The figure shows three views and two pictorial views of one solid part (mm, origin at its lowest corner). Answer the questions. A direction names the side the tool comes from. Round coordinates to 2 decimals unless told otherwise and drop trailing zeros. Write each loop counter-clockwise with the first axis right and the second up, starting at its lowest first coordinate (ties: lowest second). Pieces come first, ordered by that corner, then holes. Notation, with made-up numbers: (55, 70.5) -> (86, 70.5) arc R33 cw to (86, 106.5) -> close; hole circle Ø10 at (-21.5, 25). An arc over 180 degrees is marked (long way). One line per item, written item: value.
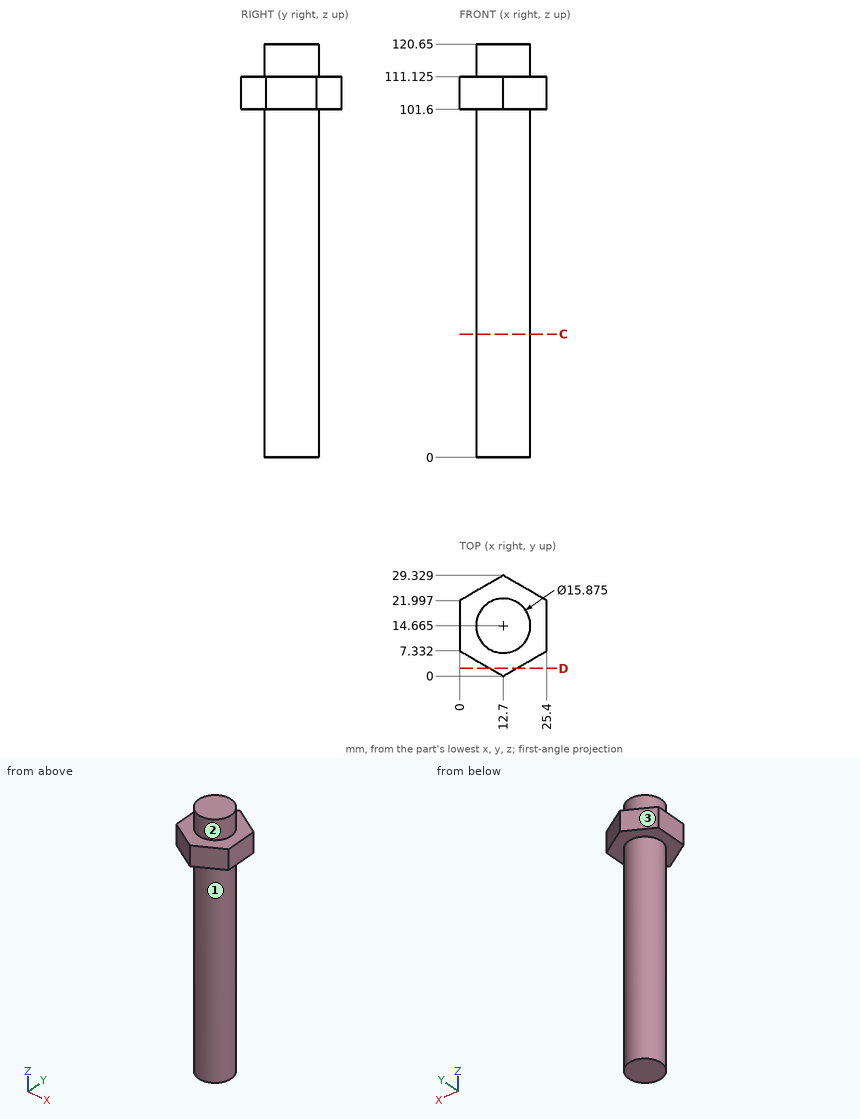
(1) Find section D-D on y = 2.25. Give the vertices of the cut face in (x, z) (1 decimal).
Reported:
outline: (8.8, 101.6) -> (16.6, 101.6) -> (16.6, 111.1) -> (8.8, 111.1) -> close
(2) Flat-ended cylindrical pins translate along their axes: pin 1 Ø7.5 at (x, y) = (18.5, 21.5) entering from -Z; pin 2 Ø1 at (x, z) = (7.5, 22.5) entering from -Y; pin 3 Ø4 at (x, y) = (4, 26) entering from -Z; pin 4 Ø2 at (y, z) = (12, 30) entering from +X. Find the tip coordinate at first contact, or state that the pin passes through.
Reported:
pin 1: stops at z = 0
pin 2: stops at y = 8.27
pin 3: stops at z = 101.6
pin 4: stops at x = 20.46
(3) A tool of negligible diameter and unlimited length cuts with its end or side. For the marked faces 1, 2 and 3, from which of +Z, -Z, +X, -X, +Y, -Y can it reach the whole face along a straight path? Write none if from no direction.
Reported:
face 1: -Z
face 2: +Z
face 3: +Z, -Z, -X, +Y
(4) Find section C-C on z = 36. Give the vertices of the cut face in (x, y) (1 decimal).
Reported:
outline: circle Ø15.9 at (12.7, 14.7)
(5) Consider probe 1 along Z at (x, y) = (19.25, 23.25) (1 decimal); probe 2 along Y at (x, z) = (13, 82); probe 3 along Y at (x, z) = (12, 33). Determine where each line is inside the solid, lowest interval first.
Reported:
probe 1: z = 101.6 to 111.1
probe 2: y = 6.73 to 22.6
probe 3: y = 6.76 to 22.57
